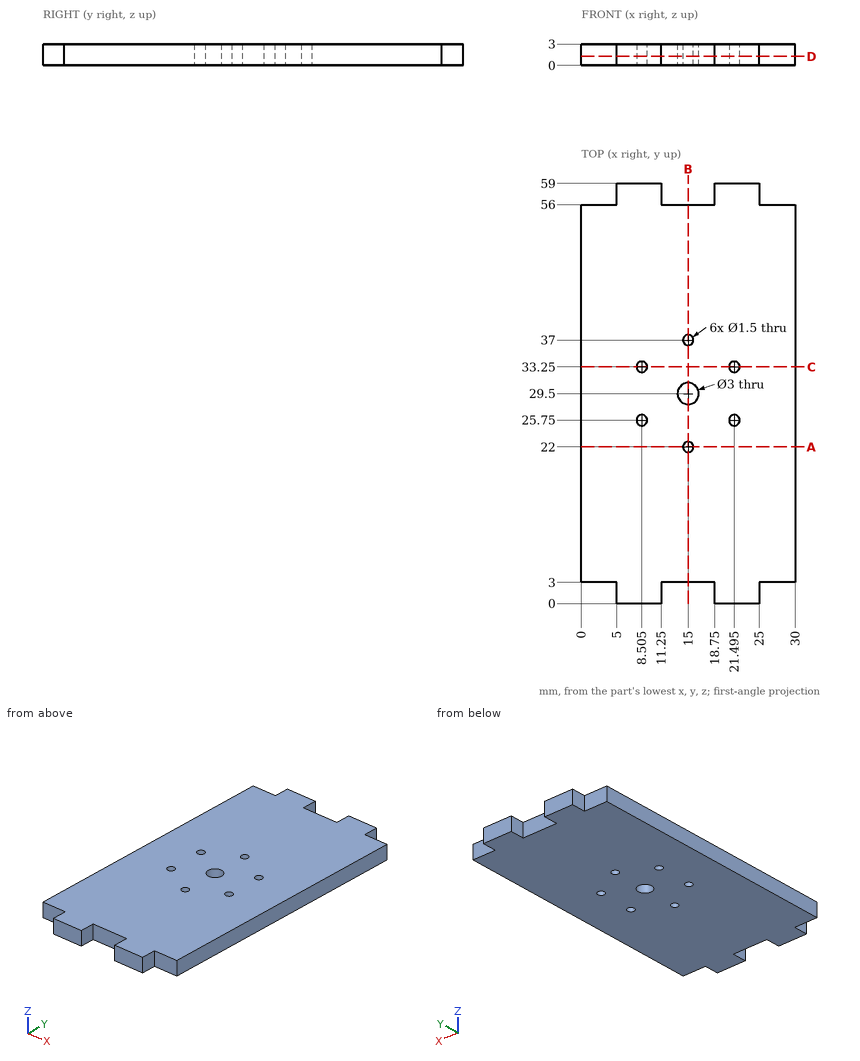
Part print with two shaded views. Sizes in mm from the minimum x, y, z corner. Round coordinates to 2 decimals unless told otherwise and drop trailing zeros. Order: outer loops, then holes, each group sorted by start corner. A loop starts at its lowest first (then second) coordinate and runs counter-clockwise, first axis right, second up. Notation, with made-up numbers: (54, 51.5) -> (59, 51.5) arc R36 ccw to (59, 86.5) -> close; hole circle Ø5 at (9, 2). An arc over 180 degrees is marked (long way). One line per question, with ' | ' between items.
Q1. Slice it at B-B (x = 15). Write the cut outline in (y, z), then the cut area to 3 significant figures.
Completed:
outline: (3, 0) -> (21.25, 0) -> (21.25, 3) -> (3, 3) -> close; (22.75, 0) -> (28, 0) -> (28, 3) -> (22.75, 3) -> close; (31, 0) -> (36.25, 0) -> (36.25, 3) -> (31, 3) -> close; (37.75, 0) -> (56, 0) -> (56, 3) -> (37.75, 3) -> close | area: 141 mm^2
Q2. Drop flat-ended pins along their axis: pin 1 (0.9 mm diameter, centred on y = 57.5, z = 1.5, fed in from -X); pin 2 (0.9 mm diameter, centred on x = 15, y = 37, fed in from +Z); pin 3 (1 mm diameter, centred on x = 3.5, z = 1.5, fed in from +Y); pin 4 (0.9 mm diameter, centred on y = 57.5, z = 1.5, fed in from +X). Give the stop position or say it passes through.
Completed:
pin 1: stops at x = 5 | pin 2: passes through | pin 3: stops at y = 56 | pin 4: stops at x = 25
Q3. Slice it at A-A (y = 22). Write the cut outline in (x, z).
Completed:
outline: (0, 0) -> (14.25, 0) -> (14.25, 3) -> (0, 3) -> close; (15.75, 0) -> (30, 0) -> (30, 3) -> (15.75, 3) -> close
Q4. Slice it at D-D (z = 1.25). Give the number of separate pieces and of enclosed holes in the cut face, then the cut area to 3 significant figures.
Completed:
separate pieces: 1 | enclosed holes: 7 | area: 1,650 mm^2
Q5. Probe probe 1 along Y at (x, z) = (15, 1.1); probe 2 along X at (y, z) = (33.25, 1.8) (1 decimal); probe 3 along Y at (x, z) = (21.5, 0.9). List the from-to ranges inside material, lowest first.
Completed:
probe 1: y = 3 to 21.25, 22.75 to 28, 31 to 36.25, 37.75 to 56 | probe 2: x = 0 to 7.8, 9.3 to 20.7, 22.2 to 30 | probe 3: y = 0 to 25, 26.5 to 32.5, 34 to 59
Q6. Slice it at C-C (y = 33.25). Write the cut outline in (x, z) (1 decimal).
Completed:
outline: (0, 0) -> (7.8, 0) -> (7.8, 3) -> (0, 3) -> close; (9.3, 0) -> (20.7, 0) -> (20.7, 3) -> (9.3, 3) -> close; (22.2, 0) -> (30, 0) -> (30, 3) -> (22.2, 3) -> close
